Part model, mm, in its own coordinate system. Face numbers are marked on the shaded views. A direction names the side the tool comes from. Give positions to 0.01 mm unless a question says otherwise; leave off trailing zeros. Order: outer loops, then holes, each group sorted by start corner. A loop starts at its lowest first (then second) coordinate and runs counter-clockwise, first axis right, second up. Notation, with made-up numbers: M 14,16 L 23,16 A31 ccw 23,44 Z; hole C 87.25,38.5 d5. An arc over 180 degrees is marked long. Write each question's results on one line, items separated by ' | '. Start each with the question number.
from build123d import *

# Parameters (mm, degrees)
F1_DEPTH = 25.4
F3_DEPTH = 25.4


with BuildPart() as f1:
    # F0 (on Right) → F1 (new body)
    with BuildSketch(Plane.YZ):
        with BuildLine():
            Line((-13.87488, 76.233894), (-34.660738, 76.233894))
            Line((-34.660738, 76.233894), (-34.660738, 0))
            Line((-34.660738, 0), (33.829767, 0))
            Line((33.829767, 0), (33.829767, 76.233894))
            Line((33.829767, 76.233894), (13.251293, 76.233894))
            Line((13.251293, 76.233894), (13.251293, 43.04883))
            ThreePointArc((13.251293, 43.04883), (-0.311793, 27.639115), (-13.87488, 43.04883))
            Line((-13.87488, 43.04883), (-13.87488, 76.233894))
        make_face()
    extrude(amount=F1_DEPTH)

    # F2 (on Top) → F3 (join)
    with BuildSketch(Plane.XY):
        with BuildLine():
            Line((0, -34.660738), (0, 34.662017))
            Line((0, 34.662017), (-38.818482, 34.662017))
            ThreePointArc((-38.818482, 34.662017), (-73.480179, 0.148866), (-39.116211, -34.660738))
            Line((-39.116211, -34.660738), (-38.520754, -34.660738))
            Line((-38.520754, -34.660738), (0, -34.660738))
        make_face()
        with BuildLine():
            Line((-38.520754, -34.660738), (-39.116211, -34.660738))
            ThreePointArc((-39.116211, -34.660738), (-38.818482, -34.662017), (-38.520754, -34.660738))
        make_face()
    extrude(amount=F3_DEPTH)


solid = f1.part
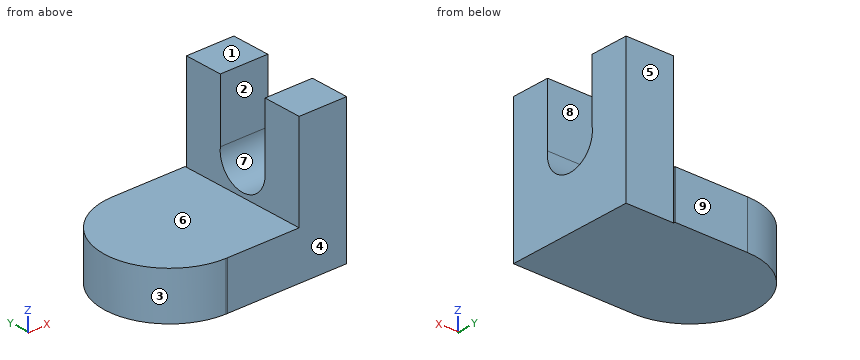
(1) Drop flat-ended pins along their axis: P1, Ø1, axis at x = -44.5, y = 12.5, coming from the -Z side; P2, Ø1, axis at x = -42, y = -12, coming from the +Z side; P3, Ø12.5, axis at x = 10, z = 54, coming from the +Y side. Give the stop position or say it passes through.
(2) Saw through at D-D on y = -17. Give the cut face in (x, z).
(3) Saw through at B-B on z = 21. Give the cut face in (x, y), plus the area to 3 significant figures.
(4) Pull direction Y, two halves, no side cores. Call the marked faces 1, 2, 3 and 4: +Y half, -Y half, draft (parallel to the pull), parting line (faces both ways), or undercut.
(5) Saw through at A-A on z = 40.5. Give the cut face in (x, y).
(6) Tool access for the marked faces 5, 6, 7, 8 and 9: list every direction of +Z, -Z, +X, -X, +Y, -Y with a clear straight run to the whole face (end or side of a thin tool).
(7) Saw through at C-C on x = 5. Give the cut face in (y, z), plus the area to 3 significant figures.
(8) Probe L1, parallel to Y at x = 7.5, z = 63.5; L2, parallel to Y at x = -10, z = 6.5; L3, parallel to X at y = 19, z = 42. List the from-to ranges inside material, lowest first.
Taken from the geometry:
1) P1: stops at z = 0 | P2: stops at z = 25.4 | P3: stops at y = 33.83
2) outline: M -69.03,0 L 25.4,0 L 25.4,76.23 L 0,76.23 L 0,25.4 L -69.03,25.4 Z
3) outline: M -39.12,-34.66 A34.65 ccw -38.52,-34.66 L 25.4,-34.66 L 25.4,33.83 L 0,33.83 L 0,34.66 L -38.82,34.66 A34.66 ccw Z | area: 6,320 mm²
4) face 1: draft | face 2: undercut | face 3: parting line | face 4: -Y half
5) outline: M 0,-34.66 L 25.4,-34.66 L 25.4,-13.96 L 0,-13.96 Z; M 0,13.34 L 25.4,13.34 L 25.4,33.83 L 0,33.83 Z
6) face 5: +Z, -Z, +X, +Y | face 6: +Z, -X, +Y, -Y | face 7: +X, -X | face 8: +Z, +X, -X | face 9: +Z, -Z, +X, -X, +Y
7) outline: M -34.66,0 L 33.83,0 L 33.83,76.23 L 13.25,76.23 L 13.25,43.05 A13.67 cw long -13.87,43.05 L -13.87,76.23 L -34.66,76.23 Z | area: 3,980 mm²
8) L1: y = -34.66 to -13.87, 13.25 to 33.83 | L2: y = -34.66 to 34.66 | L3: x = 0 to 25.4
